from build123d import *

# Parameters (mm, degrees)
SKETCH1_R           = 12.7
BOSS_EXTRUDE1_DEPTH = 12.7


with BuildPart() as part:
    # Sketch1 → Boss-Extrude1 (new body)
    with BuildSketch(Plane.XY):
        with BuildLine():
            Line((-108.405909488, -695.764543073), (50.8, -420.011818976))
            Line((50.8, -420.011818976), (50.8, 0))
            ThreePointArc((50.8, 0), (0, 50.8), (-50.8, 0))
            Line((-50.8, 0), (-50.8, -392.788181024))
            Line((-50.8, -392.788181024), (-196.394090512, -644.964543073))
            ThreePointArc((-196.394090512, -644.964543073), (-177.8, -714.358633586), (-108.405909488, -695.764543073))
        make_face()
        Circle(SKETCH1_R, mode=Mode.SUBTRACT)
        with Locations((-152.4, -670.364543073)):
            Circle(SKETCH1_R, mode=Mode.SUBTRACT)
        with Locations((0, -406.4)):
            Circle(SKETCH1_R, mode=Mode.SUBTRACT)
    extrude(amount=BOSS_EXTRUDE1_DEPTH)


solid = part.part
Can you work these out from the model? Positions are in its coordinate system, mm. A direction names the side the tool comes from. Give positions to 0.01 mm unless a question says otherwise; leave off trailing zeros. Order: outer loops, then holes, each group sorted by start corner. A loop starts at its lowest first (then second) coordinate and runs counter-clockwise, first axis right, second up. Notation, with made-up numbers: M 0.25,-28.75 L 25.25,-28.75 A16 ccw 25.25,-15.75 Z; hole C -2,-6 d7. An arc over 180 degrees is marked long. One line per item, written item: value.
Item 1: If we section it at B-B on z = 10.75: Write out the boundary of the cut face in (x, y).
Verdict:
outline: M -196.39,-644.96 A50.8 ccw -108.41,-695.76 L 50.8,-420.01 L 50.8,0 A50.8 ccw -50.8,0 L -50.8,-392.79 Z; hole C -152.4,-670.36 d25.4; hole C 0,-406.4 d25.4; hole C 0,0 d25.4
Item 2: If we mould it in two halves opening along X, with no side actions, what happens to faces 3 (the face through (-2.75, -418.8, 6.26)), 4 (the face through (-50, -330, 0)), 5 (the face through (50.8, -213, 6)), 6 (the face through (-178.76, -713.79, 6.26))? For each: pulls with the +X half, pulls with the -X half, needs draft (parallel to the pull), parting line crosses it, or undercut.
Verdict:
face 3: undercut
face 4: needs draft
face 5: pulls with the +X half
face 6: parting line crosses it
Item 3: If we section it at C-C on y = -406.4: Write out the boundary of the cut face in (x, z), and give its area (3 significant figures).
Verdict:
outline: M -58.66,0 L -12.7,0 L -12.7,12.7 L -58.66,12.7 Z; M 12.7,0 L 50.8,0 L 50.8,12.7 L 12.7,12.7 Z
area: 1,070 mm2
Item 4: Please list where these lines run through material, in increasing order: line 1 (Y direction, x = -10.5, z = 2.5); line 2 (Y direction, x = 0, z = 3.25); line 3 (X direction, y = -230, z = 7.5).
Verdict:
line 1: -526.19 to -413.54, -399.26 to -7.14, 7.14 to 49.7
line 2: -508 to -419.1, -393.7 to -12.7, 12.7 to 50.8
line 3: -50.8 to 50.8
Item 5: For faces 1 (the face through (-50, -330, 12.7)), 2 (the face through (-50.8, -194, 6)), which set-ups out of +Z, -Z, +X, -X, +Y, -Y let a thin tool reach every point of the face, with its end or its side?
Verdict:
face 1: +Z, +X, -X, +Y, -Y
face 2: +Z, -Z, -X, +Y
Item 6: If we section it at A-A on x = 0: Write out the boundary of the cut face in (y, z).
Verdict:
outline: M -508,0 L -419.1,0 L -419.1,12.7 L -508,12.7 Z; M -393.7,0 L -12.7,0 L -12.7,12.7 L -393.7,12.7 Z; M 12.7,0 L 50.8,0 L 50.8,12.7 L 12.7,12.7 Z
Item 7: For pin 1 (5 mm diameter, centred on x = -12, y = -252, fed in from -Z); pin 2 (4 mm diameter, centred on x = -87, z = 7, fed in from +Y); pin 3 (4 mm diameter, centred on y = -188, z = 6, fed in from -X); pin 4 (3 mm diameter, centred on x = -147.5, z = 9, fed in from +Y), each with a flat end and sliding along its axis, tell me the tip position at first contact or that it passes through.
Verdict:
pin 1: z = 0
pin 2: y = -452.02
pin 3: x = -50.8
pin 4: y = -557.68
Item 8: If we section it at D-D on y = -171: Write out the boundary of the cut face in (x, z), and give its area (3 significant figures).
Verdict:
outline: M -50.8,0 L 50.8,0 L 50.8,12.7 L -50.8,12.7 Z
area: 1,290 mm2
